Could you check a few things on this model? Use its own coordinates, in mm. Give positions to 0.01 mm unless a question says otherwise; leave off trailing zeros. Order: outer loops, then holes, each group sorted by start corner. A loop starts at its lowest first (then second) coordinate and runs counter-clockwise, first axis right, second up. Notation, with made-up numbers: (16, 80.25) -> (75, 80.25) arc R28 ccw to (75, 118.25) -> close; hole circle Ø11 at (81.25, 61). An arc over 180 degrees is marked (long way). Use one line per item in the form item = value. Start each with the question number.
from build123d import *

# Parameters (mm, degrees)
F1_DEPTH    = 12.7
F2_T1_DEPTH = 111.249434278


# Not quite as in the source:
# - a fillet or chamfer that OpenCascade refuses, or shapes differently, is made with other operations: its cross-section is extruded or revolved along the edge and cut away or added


with BuildPart() as f1:
    # F0 (on Front) → F1 (new body, symmetric)
    with BuildSketch(Plane.XZ):
        with BuildLine():
            Line((-55.88, 0), (-30.48, 0))
            add(Edge.make_bspline(
                [(-30.48, 0), (-27.7506317943, 14.9127226323), (-11.670826003, 16.7281851172), (0, 16.7281851172)],
                knots=[0, 0, 0, 0, 34.7687011163, 34.7687011163, 34.7687011163, 34.7687011163], degree=3))
            add(Edge.make_bspline(
                [(30.48, 0), (27.7506317943, 14.9127226323), (11.670826003, 16.7281851172), (0, 16.7281851172)],
                knots=[0, 0, 0, 0, 34.7687011163, 34.7687011163, 34.7687011163, 34.7687011163], degree=3))
            Line((30.48, 0), (55.88, 0))
            Line((55.88, 0), (55.88, 25.4))
            Line((55.88, 25.4), (-55.88, 25.4))
            Line((-55.88, 25.4), (-55.88, 0))
        make_face()
    extrude(amount=F1_DEPTH, both=True)

    # F2: fillet of radius 17.1698868556 on 4 edges, made by hand

    # F2_s2 → F2_t1 (cut)
    with BuildSketch(Plane.XY.offset(-42.924717139)):
        with BuildLine():
            ThreePointArc((55.88, 4.4698868556), (50.8510565722, -7.6710565722), (38.7101131444, -12.7))
            Line((38.7101131444, -12.7), (55.88, -12.7))
            Line((55.88, -12.7), (55.88, 4.4698868556))
        make_face()
        with BuildLine():
            ThreePointArc((55.88, -4.4698868556), (50.8510565722, 7.6710565722), (38.7101131444, 12.7))
            Line((38.7101131444, 12.7), (55.88, 12.7))
            Line((55.88, 12.7), (55.88, -4.4698868556))
        make_face()
        with BuildLine():
            ThreePointArc((-55.88, 4.4698868556), (-50.8510565722, -7.6710565722), (-38.7101131444, -12.7))
            Line((-38.7101131444, -12.7), (-55.88, -12.7))
            Line((-55.88, -12.7), (-55.88, 4.4698868556))
        make_face()
        with BuildLine():
            ThreePointArc((-55.88, -4.4698868556), (-50.8510565722, 7.6710565722), (-38.7101131444, 12.7))
            Line((-38.7101131444, 12.7), (-55.88, 12.7))
            Line((-55.88, 12.7), (-55.88, -4.4698868556))
        make_face()
    extrude(amount=F2_T1_DEPTH, mode=Mode.SUBTRACT)


solid = f1.part
(1) Imagine slicing it at B-B (x = 43). Write out the boundary of the cut face in (y, z), plus the area to 3 significant figures.
(2) Imagine slicing it at C-C (x = -43.5). Write out the boundary of the cut face in (y, z), plus the area to 3 significant figures.
(3) Imagine slicing it at A-A (z = 18). Write out the boundary of the cut face in (x, y), plus the area to 3 significant figures.
(4) I'm going to push flat-ended pins straight in: pin 1 Ø3 at (y, z) = (-4.5, 18.5) entering from +X; pin 2 Ø2 at (y, z) = (9.5, 12) entering from +X; pin 3 Ø1.5 at (x, z) = (-10.5, 13.5) entering from +Y. Where does each tip first touch, or does it pass through?
(5) Please list where these lines run through material, in increasing order: probe 1 along Y at (x, z) = (39, 2); probe 2 along X at (y, z) = (-11, 8.25); probe 3 along X at (y, z) = (4, 4.25).
Calculated:
q1.outline = (-12.16, 0) -> (12.16, 0) -> (12.16, 25.4) -> (-12.16, 25.4) -> close
q1.area = 617 mm2
q2.outline = (-12.02, 0) -> (12.02, 0) -> (12.02, 25.4) -> (-12.02, 25.4) -> close
q2.area = 611 mm2
q3.outline = (-55.29, 0) arc R17.17 ccw to (-38.71, -12.7) -> (38.71, -12.7) arc R17.17 ccw to (55.29, 0) arc R17.17 ccw to (38.71, 12.7) -> (-38.71, 12.7) arc R17.17 ccw to start
q3.area = 2,590 mm2
q4.pin_1 = 54.17
q4.pin_2 = 49.96
q4.pin_3 = through
q5.probe_1 = -12.7 to 12.7
q5.probe_2 = -46.16 to -26.78, 26.78 to 46.16
q5.probe_3 = -53.65 to -29.21, 29.21 to 53.65
